Answer from the drawing. Dimensions are ordinates in mm from the lowest x, y and z of the part. A direction names the side the tool comes from. Coordinates: 2 decimals unless noted, no trailing zeros. Write each loop counter-clockwise with the first axis right and the second up, starting at its lowest first coordinate (ties: lowest second). Pieces come first, ordered by that corner, then holes. Notation, with made-up numbers: (21.25, -31.75) - (36.25, -31.75) arc R31 ccw to (36.25, 3.25) - close; hole circle Ø10 at (75.5, 75). An arc over 180 degrees is marked (long way). Use one line per item in the form item = value. Start each with the question number.
Item 1: Determine the mould class of the marked faces 5, 6 and 7 for opening direction Z: released by +Z, released by -Z, zero draft, split by the parting line, or undercut.
Item 2: A cutting plane is placed at C-C (x = 4). Write down the section's boundary in (y, z).
Item 3: A cutting plane is placed at A-A (y = 26). Write down the section's boundary in (x, z), then the cut area to 3 significant figures.
Item 4: A cutting plane is placed at B-B (x = 65). Write down the section's boundary in (y, z).
Item 5: Given pin 1 (1.5 mm diameter, centred on y = 27.5, z = 36, fed in from -X); pin 2 (6 mm diameter, centred on y = 30.5, z = 13.5, fed in from +X); pin 3 (4 mm diameter, centred on x = 4, y = 29.5, fed in from -Z), each flat-ended and moving along its own axis, determine where each tip first touches the part or whether it passes through.
Item 6: A cutting plane is placed at D-D (z = 9.5). Write down the section's boundary in (x, y), then the cut area to 3 significant figures.
Item 7: For the marked faces 1, 2, 3 and 4, determine the directions among +Z, -Z, +X, -X, +Y, -Y from which every point of the face is accessible in a straight line to the end or side of a thin tool.
Item 8: Consider probe 1 along Y at (x, z) = (4, 1); probe 2 along X at (y, z) = (17, 31.5); probe 3 along Y at (x, z) = (20.5, 35.5). Determine where each line is inside the solid, lowest interval first.
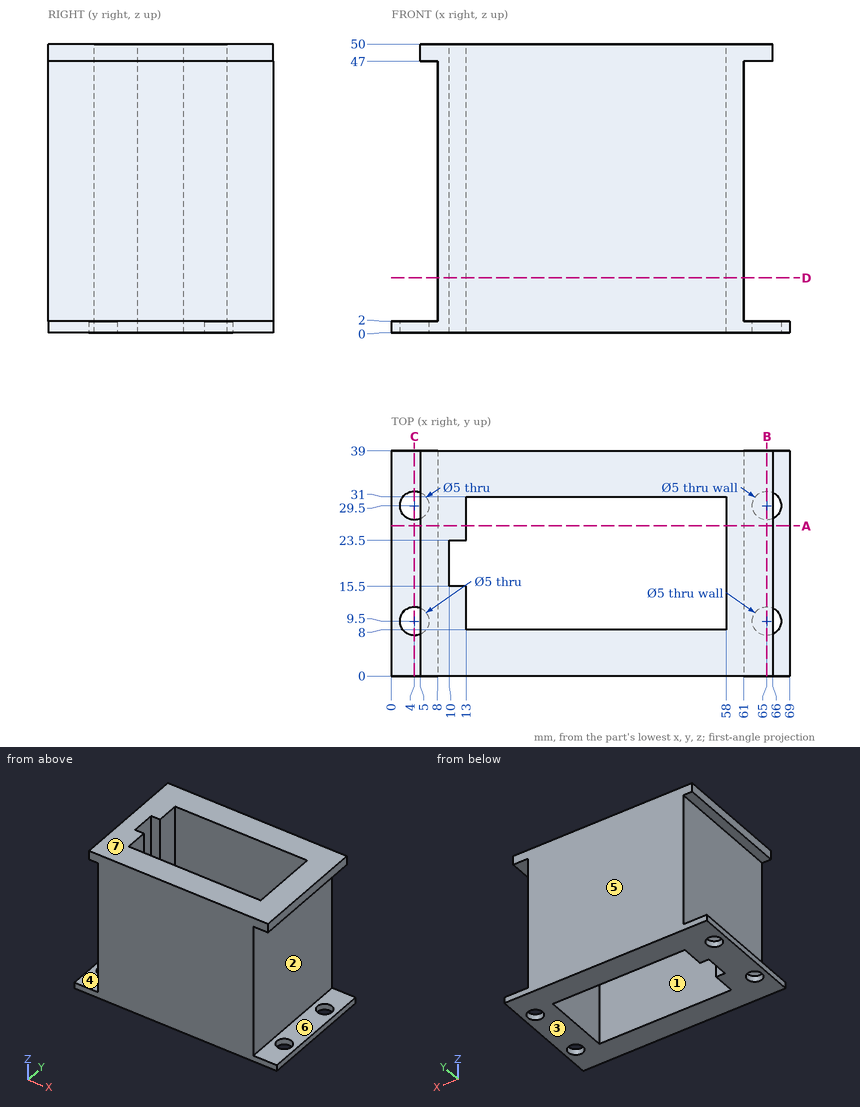
Answer:
q1.face_5 = zero draft
q1.face_6 = undercut
q1.face_7 = released by +Z
q2.outline = (0, 0) - (7, 0) - (7, 2) - (0, 2) - close; (12, 0) - (27, 0) - (27, 2) - (12, 2) - close; (32, 0) - (39, 0) - (39, 2) - (32, 2) - close
q3.outline = (0, 0) - (13, 0) - (13, 50) - (5, 50) - (5, 47) - (8, 47) - (8, 2) - (0, 2) - close; (58, 0) - (69, 0) - (69, 2) - (61, 2) - (61, 47) - (66, 47) - (66, 50) - (58, 50) - close
q3.area = 456 mm²
q4.outline = (0, 0) - (7, 0) - (7, 2) - (0, 2) - close; (0, 47) - (39, 47) - (39, 50) - (0, 50) - close; (12, 0) - (27, 0) - (27, 2) - (12, 2) - close; (32, 0) - (39, 0) - (39, 2) - (32, 2) - close
q5.pin_1 = 8
q5.pin_2 = 61
q5.pin_3 = 47
q6.outline = (8, 0) - (61, 0) - (61, 39) - (8, 39) - close; hole (10, 15.5) - (13, 15.5) - (13, 8) - (58, 8) - (58, 31) - (13, 31) - (13, 23.5) - (10, 23.5) - close
q6.area = 1,010 mm²
q7.face_1 = +Z, -Z
q7.face_2 = +X, +Y, -Y
q7.face_3 = -Z, +X, -X, +Y, -Y
q7.face_4 = -X, +Y, -Y
q8.probe_1 = 0 to 7, 12 to 27, 32 to 39
q8.probe_2 = 8 to 10, 58 to 61
q8.probe_3 = 0 to 8, 31 to 39
